Geometry: final body of the model. Coordinates: model frame, mm. Give positions to 0.01 mm unless a question says otherwise; leave off trailing zeros. Loops run counter-clockwise (first coordinate to the right, second up) from the corner with the lowest first, then second, coordinate; pieces in that order, holes last.
1. Material intervals for line 1 along X through (y, z) = (-10, 1.55); line 2 along Y through (x, z) = (12.5, 0.9); line 3 along Y through (x, z) = (14, 2.6), sorted ascending.
2. Section B-B, the plane z = 1.8. Output: boundary loops of the cut face in (x, y), then the cut area to 3 significant figures.
3. Section A-A, the plane x = 13.5. Output: boundary loops of the cut face in (y, z), then the cut area to 3 significant figures.
4. Section C-C, the plane y = -9. Output: boundary loops of the cut face in (x, z).
5. Draft query along X for faces 1 (the face through (12, -30.005, 1)), 2 (the face through (22.299, -10, 1)), 3 (the face through (14.146, -0.771, 1.479)), 4 (the face through (-11.548, 2.804, 1.479)). Return one class per face: +X half, -X half, draft (parallel to the pull), parting line (faces both ways), or undercut.
6. Section D-D, the plane x = -7. Output: boundary loops of the cut face in (y, z), then the cut area to 3 significant figures.
from build123d import *

# Parameters (mm, degrees)
SKETCH_1_R      = 2
EXTRUDE_1_DEPTH = 3


with BuildPart() as part:
    # 草图1 → 凸台-拉伸1 (new body)
    with BuildSketch(Plane.XY):
        with BuildLine():
            Line((-27.342128098, -0.00537982), (-27.342128098, -20.00537982))
            ThreePointArc((-27.342128098, -20.00537982), (-11.758458295, -22.743290911), (2.298888053, -30.00537982))
            Line((2.298888053, -30.00537982), (22.298888053, -30.00537982))
            Line((22.298888053, -30.00537982), (22.298888053, 9.99462018))
            Line((22.298888053, 9.99462018), (2.298888053, 9.99462018))
            ThreePointArc((2.298888053, 9.99462018), (-11.758458295, 2.732531272), (-27.342128098, -0.00537982))
        make_face()
        with Locations((-17.342128098, -10.00537982)):
            Circle(SKETCH_1_R, mode=Mode.SUBTRACT)
        with Locations((-7.231642467, -10.00537982)):
            Circle(SKETCH_1_R, mode=Mode.SUBTRACT)
        with Locations((12.298888053, -10.00537982)):
            Circle(SKETCH_1_R, mode=Mode.SUBTRACT)
        with Locations((12.298888053, -0.00537982)):
            Circle(SKETCH_1_R, mode=Mode.SUBTRACT)
        with Locations((12.298888053, -20.00537982)):
            Circle(SKETCH_1_R, mode=Mode.SUBTRACT)
    extrude(amount=EXTRUDE_1_DEPTH)


solid = part.part
Answers below:
1. line 1: x = -27.34 to -19.34, -15.34 to -9.23, -5.23 to 10.3, 14.3 to 22.3
1. line 2: y = -30.01 to -22, -18.02 to -12, -8.02 to -2, 1.98 to 9.99
1. line 3: y = -30.01 to -21.06, -18.95 to -11.06, -8.95 to -1.06, 1.05 to 9.99
2. outline: (-27.34, -20.01) arc R52.43 cw to (2.3, -30.01) - (22.3, -30.01) - (22.3, 9.99) - (2.3, 9.99) arc R52.43 cw to (-27.34, -0.01) - close; hole circle Ø4 at (-17.34, -10.01); hole circle Ø4 at (-7.23, -10.01); hole circle Ø4 at (12.3, -20.01); hole circle Ø4 at (12.3, -10.01); hole circle Ø4 at (12.3, -0.01)
2. area: 1,530 mm2
3. outline: (-30.01, 0) - (-21.6, 0) - (-21.6, 3) - (-30.01, 3) - close; (-18.41, 0) - (-11.6, 0) - (-11.6, 3) - (-18.41, 3) - close; (-8.41, 0) - (-1.6, 0) - (-1.6, 3) - (-8.41, 3) - close; (1.59, 0) - (9.99, 0) - (9.99, 3) - (1.59, 3) - close
3. area: 91.2 mm2
4. outline: (-27.34, 0) - (-19.07, 0) - (-19.07, 3) - (-27.34, 3) - close; (-15.61, 0) - (-8.96, 0) - (-8.96, 3) - (-15.61, 3) - close; (-5.5, 0) - (10.57, 0) - (10.57, 3) - (-5.5, 3) - close; (14.03, 0) - (22.3, 0) - (22.3, 3) - (14.03, 3) - close
5. face 1: draft
5. face 2: +X half
5. face 3: undercut
5. face 4: -X half
6. outline: (-24.61, 0) - (-11.99, 0) - (-11.99, 3) - (-24.61, 3) - close; (-8.02, 0) - (4.6, 0) - (4.6, 3) - (-8.02, 3) - close
6. area: 75.7 mm2
